Job drawing, mm, ordinate dimensions from the low corner. One solid piece. A direction names the side the tool comes from. Round coordinates to 2 decimals unless told otherwise and drop trailing zeros. Write each loop counter-clockwise with the first axis right and the second up, starting at its lowest first coordinate (ties: lowest second). Pieces come first, ordered by that corner, then holes. Notation, with made-up numbers: (-18.5, 22) - (39.5, 22) arc R14 cw to (39.5, 26) - close; hole circle Ø3 at (16, 35). An arc over 180 degrees is marked (long way). Write each question's results on one line, items separated by ' | '.
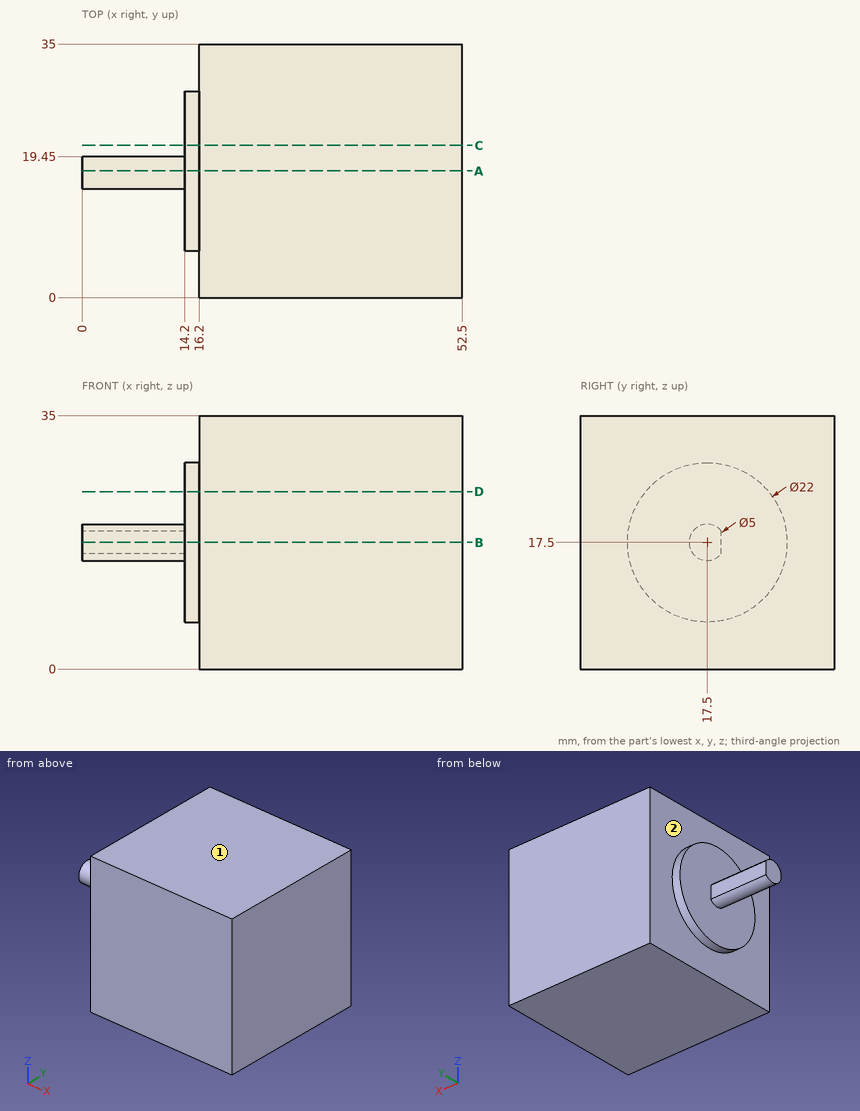
(1) Drill centre lines: probe 1 along X at (y, z) = (16, 5); probe 2 along X at (y, z) = (7, 17); probe 3 along Y at (x, z) = (8.5, 15.5). Where is each one in solid material? Low to high. Write a range as [from, to].
Worked answers:
probe 1: x = [16.2, 52.5] | probe 2: x = [14.2, 52.5] | probe 3: y = [16, 19]
(2) Slice it at B-B, the plane z = 17.5. Write the cut outline in (x, y).
Worked answers:
outline: (0, 15) - (14.2, 15) - (14.2, 6.5) - (16.2, 6.5) - (16.2, 0) - (52.5, 0) - (52.5, 35) - (16.2, 35) - (16.2, 28.5) - (14.2, 28.5) - (14.2, 19.45) - (0, 19.45) - close
(3) Slice it at C-C, the plane y = 21. Write the cut outline in (x, z), and give its area (3 significant figures).
Worked answers:
outline: (14.2, 7.07) - (16.2, 7.07) - (16.2, 0) - (52.5, 0) - (52.5, 35) - (16.2, 35) - (16.2, 27.93) - (14.2, 27.93) - close | area: 1,310 mm2
(4) Slice it at A-A, the plane y = 17.5. Write the cut outline in (x, z), and give its area (3 significant figures).
Worked answers:
outline: (0, 15) - (14.2, 15) - (14.2, 6.5) - (16.2, 6.5) - (16.2, 0) - (52.5, 0) - (52.5, 35) - (16.2, 35) - (16.2, 28.5) - (14.2, 28.5) - (14.2, 20) - (0, 20) - close | area: 1,390 mm2
(5) Slice it at D-D, the plane z = 24.5. Write the cut outline in (x, y), and give its area (3 significant figures).
Worked answers:
outline: (14.2, 9.01) - (16.2, 9.01) - (16.2, 0) - (52.5, 0) - (52.5, 35) - (16.2, 35) - (16.2, 25.99) - (14.2, 25.99) - close | area: 1,300 mm2
(6) Tool access for the marked faces 1 and 2: list every direction of +Z, -Z, +X, -X, +Y, -Y with a clear straight run to the whole face (end or side of a thin tool).
Worked answers:
face 1: +Z, +X, -X, +Y, -Y | face 2: -X
(7) Flat gauge pins, fed straight in: pin 1 Ø1.6 at (x, z) = (5, 18) entering from +Y; pin 2 Ø12 at (y, z) = (11.5, 27.5) entering from -X. Where does each tip first touch, or does it go through?
Worked answers:
pin 1: stops at y = 19.45 | pin 2: stops at x = 14.2
